Source: three-view drawing plus pictorial views. Frame: mm from the lowest corner of the part. A direction names the side the tool comes from. Round coordinates to 2 decimals unless told otherwise and drop trailing zeros. Loops run counter-clockwise (first coordinate to the right, second up) from the corner with the lowest first, then second, coordinate; pieces in that order, holes last. Notation, with made-up numbers: M 23,72.5 L 53,72.5 A24 cw 53,91.5 Z; hole C 50,43 d4. An arc over 180 degrees is marked long. Return JSON: item names as keys, results as strings. Group by question number.
1) Section D-D (z = 25.5). Output: boundary loops of the cut face in (x, y) (1 decimal).
2) Contact query for flat-ended pins moving along their axis: P1, Ø4, axis at x = 16.5, z = 8.5, coming from the +Y side (1 decimal); P2, Ø4, axis at x = 37.5, z = 16.5, coming from the +Y side (1 decimal); P3, Ø6, axis at x = 31.5, y = 8, coming from the -Z side. Output: stop coordinate, or through.
3) Material intervals for line 1 (Z direction, x = 21, y = 29); line 2 (X direction, y = 21, z = 22), sorted ascending. Write a range as from..to.
4) Mould query, pull axis Z, two halves, no side actions, for the marked faces 1, 2 and 3. Classes: +Z half, -Z half, draft (parallel to the pull), parting line (faces both ways), or undercut.
5) Access query for the marked faces 4 and 5. Directions: +Z, -Z, +X, -X, +Y, -Y. A direction counts if a zero-diameter tool reaches every point of the face in a straight line with its end or side. Return the directions, or none.
6) Section C-C (z = 20.25). Output: boundary loops of the cut face in (x, y), plus the area to 3 significant figures.
7) Section A-A (y = 20.9). Output: boundary loops of the cut face in (x, z).
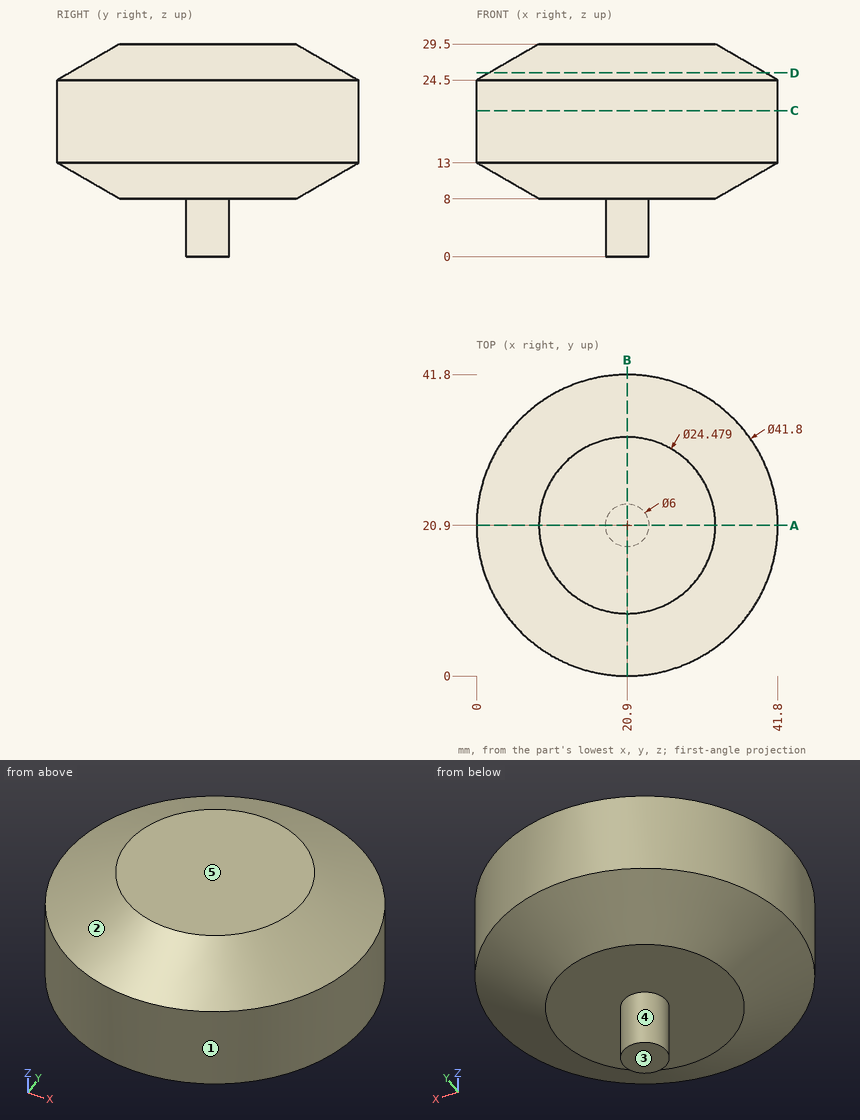
Returned:
{
 "1": {"outline": "C 20.9,20.9 d38.3"},
 "2": {"P1": "stops at y = 36.9", "P2": "stops at y = 35.9", "P3": "stops at z = 8.84"},
 "3": {"line 1": "z = 8..29.5", "line 2": "x = 0..41.8"},
 "4": {"face 1": "draft", "face 2": "+Z half", "face 3": "-Z half"},
 "5": {"face 4": "-Z", "face 5": "+Z, +X, -X, +Y, -Y"},
 "6": {"outline": "C 20.9,20.9 d41.8", "area": "1,370 mm^2"},
 "7": {"outline": "M 0,13 L 8.66,8 L 17.9,8 L 17.9,0 L 23.9,0 L 23.9,8 L 33.14,8 L 41.8,13 L 41.8,24.5 L 33.14,29.5 L 8.66,29.5 L 0,24.5 Z"}
}
